```python
from build123d import *

# Parameters (mm, degrees)
SKETCH_1_W          = 32.677388302
SKETCH_1_H          = 15.432977872
EXTRUDE_1_DEPTH     = 25
SKETCH_2_R          = 1.25
CUT_EXTRUDE_1_DEPTH = 26
SKETCH_3_R          = 6
EXTRUDE_2_DEPTH     = 15.432978
SKETCH_4_R          = 4
CUT_EXTRUDE_2_DEPTH = 16.432978
EXTRUDE_3_DEPTH     = 15.432978
SKETCH_6_W          = 6
SKETCH_6_H          = 8.481168663
EXTRUDE_4_DEPTH     = 15.432978
SKETCH_8_W          = 3
SKETCH_8_H          = 25.378391716
CUT_EXTRUDE_5_DEPTH = 16.432978
SKETCH_9_R          = 1.5
CUT_EXTRUDE_6_DEPTH = 20.338694151
FILLET_1_R          = 2
FILLET_2_R          = 2


with BuildPart() as part:
    # Sketch 1 → Extrude 1 (new body)
    with BuildSketch(Plane.XY):
        with Locations((-3.726697353, 26.358574689)):
            Rectangle(SKETCH_1_W, SKETCH_1_H)
    extrude(amount=-EXTRUDE_1_DEPTH)

    # Sketch 2 → Cut-Extrude 1 (cut, through all)
    with BuildSketch(Plane.XY):
        with Locations((-12.726697353, 26.358574689)):
            Circle(SKETCH_2_R)
        with Locations((5.273302647, 26.358574689)):
            Circle(SKETCH_2_R)
    extrude(amount=-CUT_EXTRUDE_1_DEPTH, mode=Mode.SUBTRACT)



with BuildPart() as body_2:
    # Sketch 3 → Extrude 2 (new body)
    with BuildSketch(Plane.XZ.offset(-18.642085753)):
        with Locations((-3.726697353, 6)):
            Circle(SKETCH_3_R)
    extrude(amount=-EXTRUDE_2_DEPTH)

    # Sketch 4 → Cut-Extrude 2 (cut, through all)
    with BuildSketch(Plane.XZ.offset(-18.642085753)):
        with Locations((-3.726697353, 6)):
            Circle(SKETCH_4_R)
    extrude(amount=-CUT_EXTRUDE_2_DEPTH, mode=Mode.SUBTRACT)


with BuildPart() as part_1:
    add(part.part)

    add(body_2.part)  # Extrude 3 merges body 2
    # Sketch 5 → Extrude 3 (add)
    with BuildSketch(Plane.XZ.offset(-18.642085753)):
        Polygon((-3.726697353, 0), (-9.726697353, 6), (-9.726697353, 0), align=None)
        Polygon((2.273302647, 6), (-3.726697353, 0), (2.273302647, 0), align=None)
    extrude(amount=-EXTRUDE_3_DEPTH)

    # Sketch 6 → Extrude 4 (add)
    with BuildSketch(Plane.XZ.offset(-18.642085753)):
        with Locations((-3.726697353, 14.240584332)):
            Rectangle(SKETCH_6_W, SKETCH_6_H)
    extrude(amount=-EXTRUDE_4_DEPTH)

    # Sketch 8 → Cut-Extrude 5 (cut, through all)
    with BuildSketch(Plane.XZ.offset(-18.642085753)):
        with Locations((-3.726697353, 18.689195858)):
            Rectangle(SKETCH_8_W, SKETCH_8_H)
    extrude(amount=-CUT_EXTRUDE_5_DEPTH, mode=Mode.SUBTRACT)

    # Sketch 9 → Cut-Extrude 6 (cut, through all)
    with BuildSketch(Plane(origin=(-0.726697353, 0, 0), x_dir=(0, 0, -1), z_dir=(1, 0, 0))):
        with Locations((-14.838660543, 26.358574689)):
            Circle(SKETCH_9_R)
    extrude(amount=-CUT_EXTRUDE_6_DEPTH, mode=Mode.SUBTRACT)

    # Fillet 1
    fillet_1_edges = [part_1.edges().sort_by_distance(p)[0] for p in [
        (12.611996798, 18.642085753, -12.5),
        (-20.065391504, 18.642085753, -12.5),
        (-20.065391504, 34.075063625, -12.5),
        (12.611996798, 34.075063625, -12.5),
    ]]
    fillet(fillet_1_edges, radius=FILLET_1_R)

    # Fillet 2
    fillet_2_edges = [part_1.edges().sort_by_distance(p)[0] for p in [
        (-1.476697353, 18.642085753, 18.481168663),
        (-1.476697353, 34.075063753, 18.481168663),
        (-5.976697353, 34.075063753, 18.481168663),
        (-5.976697353, 18.642085753, 18.481168663),
    ]]
    fillet(fillet_2_edges, radius=FILLET_2_R)


solid = part_1.part
```
Can you work these out from the model? Positions are in its coordinate system, mm. A direction names the side the tool comes from. Give positions to 0.01 mm unless a question says otherwise; leave off trailing zeros. Loops run counter-clockwise (first coordinate to the right, second up) from the corner with the lowest first, then second, coordinate; pieces in that order, holes last. Notation, with made-up numbers: M 59,-19.5 L 87,-19.5 A38 cw 87,19.5 Z; hole C -0.75,-16.75 d11. An arc over 180 degrees is marked long. Answer in a Markdown table with one row per item.
1. Suppose I cut it at A-A on y = 29.75. Write out the boundary of the cut face in (x, z).
Taken from the geometry:
| item | result |
|---|---|
| outline | M -20.07,-25 L 12.61,-25 L 12.61,0 L 2.27,0 L 2.27,6 A6 ccw -0.73,11.2 L -0.73,18.48 L -2.23,18.48 L -2.23,9.71 A4 cw long -5.23,9.71 L -5.23,18.48 L -6.73,18.48 L -6.73,11.2 A6 ccw -9.73,6 L -9.73,0 L -20.07,0 Z |
2. Which directions (+Z, -Z, +X, -X, +Y, -Y) give clear straight access to the entire face, cutting with the end or side of a thin tool? Please do faces 1 (the flat face through (-2.227, 26, 13)), 2 (the flat face through (7, 26, 0)), 3 (the cylindrical face through (-19.46, 19.21, -12.68)), 4 (the flat face through (-15, 26, 0)).
Taken from the geometry:
| item | result |
|---|---|
| face 1 | +Z, +Y, -Y |
| face 2 | +Z, +X, +Y, -Y |
| face 3 | +Z, -Z, -X, -Y |
| face 4 | +Z, -X, +Y, -Y |
3. Suppose I cut it at B-B on z = 7. Write out the boundary of the cut face in (x, y).
Taken from the geometry:
| item | result |
|---|---|
| outline | M -9.64,18.64 L -7.6,18.64 L -7.6,34.08 L -9.64,34.08 Z; M 0.15,18.64 L 2.19,18.64 L 2.19,34.08 L 0.15,34.08 Z |
4. Thinking about a two-plate mould opening in X: for faces 5 (the cylindrical face through (-5.966, 33.474, 17.911)), 6 (the cylindrical face through (-12.05, 27.41, -12.32)), 7 (the cylindrical face through (12.042, 33.474, -12.675)), 8 (the flat face through (-9.727, 26, 3)), which applies, released by +X, released by -X, zero draft, split by the parting line, or undercut?
Taken from the geometry:
| item | result |
|---|---|
| face 5 | zero draft |
| face 6 | undercut |
| face 7 | released by +X |
| face 8 | released by -X |
5. If I drill on line 1 along X through (y, z) = (28.5, 6); line 2 along Z through (x, y) = (-6, 27.25); line 3 along Z through (x, y) = (-10.5, 20.25), over which ranges is the centre line in solid material (lowest first)?
Taken from the geometry:
| item | result |
|---|---|
| line 1 | x = -9.73 to -7.73, 0.27 to 2.27 |
| line 2 | z = -25 to 2.71, 9.29 to 13.63, 16.05 to 18.48 |
| line 3 | z = -25 to 0 |
6. For pin 1 Ø5 at (y, z) = (25, 3.5) entering from +X; pin 2 Ø5 at (y, z) = (26.5, 3.5) entering from -X; pin 3 Ø8.5 at (x, y) = (5, 25) entering from +Z, each with a flat end and sliding along its axis, tell me the tip position at first contact or that it passes through.
Taken from the geometry:
| item | result |
|---|---|
| pin 1 | stops at x = 2.27 |
| pin 2 | stops at x = -9.73 |
| pin 3 | stops at z = 9.99 |
7. Suppose I cut it at C-C on x = 6. Write out the boundary of the cut face in (y, z), plus the area to 3 significant figures.
Taken from the geometry:
| item | result |
|---|---|
| outline | M 18.64,-25 L 25.34,-25 L 25.34,0 L 18.64,0 Z; M 27.38,-25 L 34.08,-25 L 34.08,0 L 27.38,0 Z |
| area | 335 mm² |
8. Suppose I cut it at D-D on z = -1. Write out the boundary of the cut face in (x, y), plus the area to 3 significant figures.
Taken from the geometry:
| item | result |
|---|---|
| outline | M -20.07,20.64 A2 ccw -18.07,18.64 L 10.61,18.64 A2 ccw 12.61,20.64 L 12.61,32.08 A2 ccw 10.61,34.08 L -18.07,34.08 A2 ccw -20.07,32.08 Z; hole C -12.73,26.36 d2.5; hole C 5.27,26.36 d2.5 |
| area | 491 mm² |
